```python
from build123d import *

# Parameters (mm, degrees)
SKETCH1_R           = 1.985
BOSS_EXTRUDE1_DEPTH = 17


with BuildPart() as part:
    # Sketch1 → Boss-Extrude1 (new body)
    with BuildSketch(Plane(origin=(0, 0, 0), x_dir=(1, 0, 0), z_dir=(0, 1, 0))):
        with BuildLine():
            ThreePointArc((-0.993994068, 5.409433962), (-1.881110788, 5.168309414), (-2.715673494, 4.782793898))
            ThreePointArc((-2.715673494, 4.782793898), (-2.806527228, 4.672511809), (-2.800603755, 4.529748184))
            ThreePointArc((-2.800603755, 4.529748184), (-3.021101766, 3.600408883), (-3.974611392, 3.544638808))
            ThreePointArc((-3.974611392, 3.544638808), (-4.114177517, 3.575262934), (-4.238560759, 3.504939756))
            ThreePointArc((-4.238560759, 3.504939756), (-4.763139721, 2.75), (-5.154647247, 1.918231415))
            ThreePointArc((-5.154647247, 1.918231415), (-5.153357284, 1.775350778), (-5.057052951, 1.669795032))
            ThreePointArc((-5.057052951, 1.669795032), (-4.628596439, 0.816146435), (-5.323178877, 0.160519906))
            ThreePointArc((-5.323178877, 0.160519906), (-5.44977754, 0.094267971), (-5.499857764, -0.039554715))
            ThreePointArc((-5.499857764, -0.039554715), (-5.416442642, -0.955064977), (-5.181704266, -1.843892867))
            ThreePointArc((-5.181704266, -1.843892867), (-5.088874194, -1.952516612), (-4.947250869, -1.971473774))
            ThreePointArc((-4.947250869, -1.971473774), (-4.070319398, -2.35), (-4.180971805, -3.298708045))
            ThreePointArc((-4.180971805, -3.298708045), (-4.235366084, -3.430836023), (-4.187710197, -3.565541096))
            ThreePointArc((-4.187710197, -3.565541096), (-3.535331853, -4.213244437), (-2.78418427, -4.743239183))
            ThreePointArc((-2.78418427, -4.743239183), (-2.643250312, -4.76677978), (-2.522575122, -4.69026809))
            ThreePointArc((-2.522575122, -4.69026809), (-1.607494674, -4.416555318), (-1.082441559, -5.21443384))
            ThreePointArc((-1.082441559, -5.21443384), (-1.039179767, -5.350613712), (-0.916086488, -5.423171171))
            ThreePointArc((-0.916086488, -5.423171171), (0, -5.5), (0.916086488, -5.423171171))
            ThreePointArc((0.916086488, -5.423171171), (1.039179767, -5.350613712), (1.082441559, -5.21443384))
            ThreePointArc((1.082441559, -5.21443384), (1.607494674, -4.416555318), (2.522575122, -4.69026809))
            ThreePointArc((2.522575122, -4.69026809), (2.643250312, -4.76677978), (2.78418427, -4.743239183))
            ThreePointArc((2.78418427, -4.743239183), (3.535331853, -4.213244437), (4.187710197, -3.565541096))
            ThreePointArc((4.187710197, -3.565541096), (4.235366084, -3.430836023), (4.180971805, -3.298708045))
            ThreePointArc((4.180971805, -3.298708045), (4.070319398, -2.35), (4.947250869, -1.971473774))
            ThreePointArc((4.947250869, -1.971473774), (5.088874194, -1.952516612), (5.181704266, -1.843892867))
            ThreePointArc((5.181704266, -1.843892867), (5.416442642, -0.955064977), (5.499857764, -0.039554715))
            ThreePointArc((5.499857764, -0.039554715), (5.44977754, 0.094267971), (5.323178877, 0.160519906))
            ThreePointArc((5.323178877, 0.160519906), (4.628596439, 0.816146435), (5.057052951, 1.669795032))
            ThreePointArc((5.057052951, 1.669795032), (5.153357284, 1.775350778), (5.154647247, 1.918231415))
            ThreePointArc((5.154647247, 1.918231415), (4.763139721, 2.75), (4.238560759, 3.504939756))
            ThreePointArc((4.238560759, 3.504939756), (4.114177517, 3.575262934), (3.974611392, 3.544638808))
            ThreePointArc((3.974611392, 3.544638808), (3.021101766, 3.600408883), (2.800603755, 4.529748184))
            ThreePointArc((2.800603755, 4.529748184), (2.806527228, 4.672511809), (2.715673494, 4.782793898))
            ThreePointArc((2.715673494, 4.782793898), (1.881110788, 5.168309414), (0.993994068, 5.409433962))
            ThreePointArc((0.993994068, 5.409433962), (0.85350811, 5.383352635), (0.766279064, 5.270181818))
            ThreePointArc((0.766279064, 5.270181818), (0, 4.7), (-0.766279064, 5.270181818))
            ThreePointArc((-0.766279064, 5.270181818), (-0.85350811, 5.383352635), (-0.993994068, 5.409433962))
        make_face()
        with Locations(Location((0, 0, 0), (0, 0, 270))):
            Circle(SKETCH1_R, mode=Mode.SUBTRACT)
    extrude(amount=BOSS_EXTRUDE1_DEPTH)


solid = part.part
```
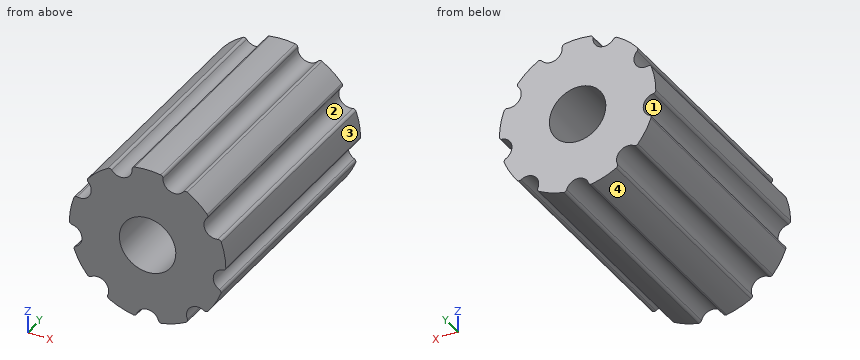
Build history of the part. All positions in model axes, mm. Face numbers are marked on the shaded views. Give positions to 0.01 mm unless a question says otherwise; leave off trailing zeros. Loops run counter-clockwise (first coordinate to the right, second up) from the corner with the lowest first, then second, coordinate; pieces in that order, holes last. Notation, with made-up numbers: (69.5, -10) -> (107.5, -10) arc R21 ccw to (107.5, 6) -> close; hole circle Ø10 at (-28.75, -2.5). An arc over 180 degrees is marked (long way). One line per question, with ' | ' between items. Start each with the question number.
1) Cut at B-B (z = 1). Give the cut face in (x, y).
2) Pin check, flat tips, straight feed: pin 1 (1.5 mm diameter, centred on y = 4.5, z = 4, fed in from -X); pin 2 (4 mm diameter, centred on x = -4.5, y = 11.5, fed in from -Z); pin 3 (1 mm diameter, centred on y = 10.5, z = -1.5, fed in from +X); pin 4 (3.5 mm diameter, centred on x = 0, z = 0, fed in from +Y). Stop position of each tip, or through.
3) Cut at D-D (z = -4). Give the cut face in (x, y), plus the area to 3 significant figures.
4) Cut at C-C (x = 3.75). Give the cut face in (y, z).
5) Cut at A-A (x = 0). Give the cut face in (y, z) (3 decimals).
6) Probe L1, parallel to X at y = 10.75, z = 0 (3 decimals); L2, parallel to X at y = 11.5, z = -3.5; L3, parallel to Z at x = 1.25, y = 2.75. List the from-to ranges inside material, lowest first.
7) Two-plate mould, pull along Z, no slides. Class the marked faces 1, 2, 3 and 4: released by +Z, released by -Z, zero draft, split by the parting line, or undercut.
Return value:
1) outline: (-5.41, 0) -> (-1.71, 0) -> (-1.71, 17) -> (-5.41, 17) -> close; (1.71, 0) -> (5.41, 0) -> (5.41, 17) -> (1.71, 17) -> close
2) pin 1: x = -4.24 | pin 2: z = -4.9 | pin 3: x = 5.17 | pin 4: through
3) outline: (-2.76, 0) -> (2.76, 0) -> (2.76, 17) -> (-2.76, 17) -> close | area: 94.0 mm^2
4) outline: (0, -3.44) -> (17, -3.44) -> (17, 4.02) -> (0, 4.02) -> close
5) outline: (0, -4.7) -> (17, -4.7) -> (17, -1.985) -> (0, -1.985) -> close; (0, 1.985) -> (17, 1.985) -> (17, 5.5) -> (0, 5.5) -> close
6) L1: -5.496 to -1.985, 1.985 to 5.496 | L2: -4.24 to -3.9, -3.17 to 3.17, 3.9 to 4.24 | L3: -5.36 to -1.54, 1.54 to 4.68
7) face 1: undercut | face 2: undercut | face 3: released by +Z | face 4: released by -Z
